from build123d import *

# Parameters (mm, degrees)
BOSS_EXTRUDE4_DEPTH = 4
SKETCH3_R           = 20
BOSS_EXTRUDE5_DEPTH = 40
SKETCH4_W           = 38.356352869
SKETCH4_H           = 36.352662793
SKETCH4_W_2         = 41.648129421
SKETCH4_H_2         = 27.192936736
SKETCH4_W_3         = 57.677650023
SKETCH4_H_3         = 26.910385372
SKETCH4_W_4         = 38.070111429
SKETCH4_H_4         = 39.361887981
CUT_EXTRUDE5_DEPTH  = 40
SKETCH7_R           = 0.75
CUT_EXTRUDE6_DEPTH  = 5


with BuildPart() as part:
    # Sketch2 → Boss-Extrude4 (new body)
    with BuildSketch(Plane(origin=(0, 0, 0), x_dir=(1, 0, 0), z_dir=(0, 1, 0))):
        with BuildLine():
            Line((0, 95), (0, 0))
            Line((0, 0), (110, 0))
            Line((110, 0), (110, 95))
            Line((110, 95), (72.04868569, 95))
            ThreePointArc((72.04868569, 95), (55, 104.543312367), (37.95131431, 95))
            Line((37.95131431, 95), (0, 95))
        make_face()
    extrude(amount=BOSS_EXTRUDE4_DEPTH)

    # Sketch3 → Boss-Extrude5 (add)
    with BuildSketch(Plane(origin=(0, 4, 0), x_dir=(1, 0, 0), z_dir=(0, 1, 0))):
        with Locations((55, 82.97105055)):
            Circle(SKETCH3_R)
    extrude(amount=BOSS_EXTRUDE5_DEPTH)

    # Sketch4 → Cut-Extrude5 (cut)
    with BuildSketch(Plane(origin=(0, 44, 0), x_dir=(1, 0, 0), z_dir=(0, 1, 0))):
        with Locations((33.821823565, 62.794719153)):
            Rectangle(SKETCH4_W, SKETCH4_H)
        with Locations((32.17593529, 98.567518918)):
            Rectangle(SKETCH4_W_2, SKETCH4_H_2)
        with Locations((85.838825012, 98.426243236)):
            Rectangle(SKETCH4_W_3, SKETCH4_H_3)
        with Locations((76.035055715, 61.29010656)):
            Rectangle(SKETCH4_W_4, SKETCH4_H_4)
    extrude(amount=-CUT_EXTRUDE5_DEPTH, mode=Mode.SUBTRACT)

    # Sketch7 → Cut-Extrude6 (cut, through all)
    with BuildSketch(Plane(origin=(0, 4, 0), x_dir=(1, 0, 0), z_dir=(0, 1, 0))):
        with Locations((45.324714989, 89.67105055)):
            Circle(SKETCH7_R)
        with Locations((48.261379546, 92.386930017)):
            Circle(SKETCH7_R)
        with Locations((61.738620454, 92.386930017)):
            Circle(SKETCH7_R)
        with Locations((64.675285011, 89.67105055)):
            Circle(SKETCH7_R)
        with Locations((64.675285011, 76.27105055)):
            Circle(SKETCH7_R)
        with Locations((61.738620454, 73.555171083)):
            Circle(SKETCH7_R)
        with Locations((48.261379546, 73.555171083)):
            Circle(SKETCH7_R)
        with Locations((45.324714989, 76.27105055)):
            Circle(SKETCH7_R)
    extrude(amount=-CUT_EXTRUDE6_DEPTH, mode=Mode.SUBTRACT)


solid = part.part
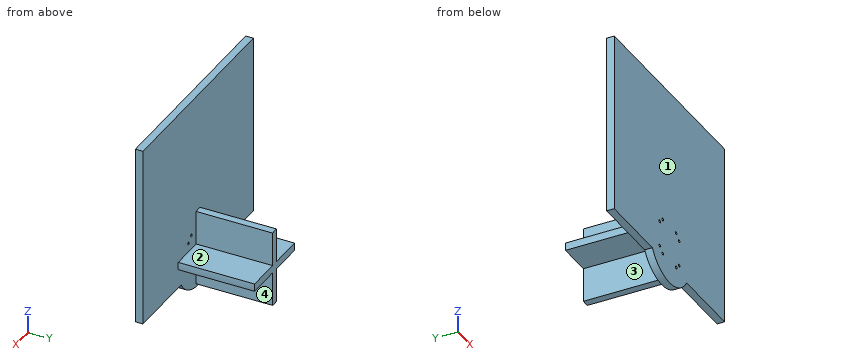
Check sheet for the modelled part. Datum: model origin and axes. Units: mm. Face numbers are marked on the shaded views. A direction names the side the tool comes from. Round coordinates to 2 decimals unless told otherwise and drop trailing zeros. Loops run counter-clockwise (first coordinate to the right, second up) from the corner with the lowest first, then second, coordinate; pieces in that order, holes last. Notation, with made-up numbers: M 78,77 L 135,77 A27 ccw 135,105 Z; hole C 80.5,-8 d5. An arc over 180 degrees is marked long. One line per question, with ' | ' between items. Start each with the question number.
Item 1: Section check D-D (x = 90.5). Record the boundary of the cut face in (y, z), and give its area (3 significant figures).
Item 2: Gauge pin test, flat ends, axial feed: pin 1 Ø1 at (x, z) = (65.5, -23.5) entering from +Y; pin 2 Ø0.9 at (x, z) = (64.68, -89.67) entering from -Y; pin 3 Ø5 at (x, y) = (44, 5) entering from -Z; pin 4 Ø9 at (x, y) = (43.5, 22.5) entering from -Z. Record the tip position at first contact, or that the pin passes through.
Item 3: Scan lines: probe 1 along Y at (x, z) = (82.5, -29); probe 2 along Z at (x, y) = (65.5, 26); probe 3 along X at (y, z) = (15.5, -72.5). Record each from-to range of solid material in increasing order.
Item 4: Section check C-C (z = -83). Record the boundary of the cut face in (x, y), and give its area (3 significant figures).
Item 5: Section check A-A (y = 20). Record the boundary of the cut face in (x, z), and give its area (3 significant figures).
Item 6: Section check B-B (x = 51). Record the boundary of the cut face in (y, z), and give its area (3 significant figures).
Item 7: Set-up check for the marked faces 1, 2, 3 and 4: record each of +Z, -Z, +X, -X, +Y, -Y from which the full face is reachable in a straight line by a thin tool's end or side.
Worked out:
1) outline: M 0,-95 L 4,-95 L 4,0 L 0,0 Z | area: 380 mm^2
2) pin 1: y = 4 | pin 2: through | pin 3: z = -102.55 | pin 4: z = -84.97
3) probe 1: 0 to 4 | probe 2: -84.97 to -80.97 | probe 3: 53 to 57
4) outline: M 0,0 L 110,0 L 110,4 L 75,4 L 75,44 L 35,44 L 35,4 L 0,4 Z | area: 2,040 mm^2
5) outline: M 35.1,-84.97 L 53,-84.97 L 53,-102.87 A20 ccw 57,-102.87 L 57,-84.97 L 74.9,-84.97 A20 ccw 74.9,-80.97 L 57,-80.97 L 57,-63.07 A20 ccw 53,-63.07 L 53,-80.97 L 35.1,-80.97 A20 ccw Z | area: 303 mm^2
6) outline: M 0,-104.14 L 4,-104.14 L 4,-84.97 L 44,-84.97 L 44,-80.97 L 4,-80.97 L 4,0 L 0,0 Z | area: 577 mm^2
7) face 1: +Z, -Z, +X, -X, -Y | face 2: +Z, +X, +Y | face 3: -Z, -X, +Y | face 4: -Z, +X, +Y
